Can you work these out from the drawing? Everything is in mm from the part's minimum corner. A direction names the side the tool comes from. Coordinates: 2 decimals unless noted, no trailing zeros. Loops run counter-clockwise (first coordinate to the right, second up) from the corner with the lowest first, then second, coordinate; pieces in that order, holes last. Notation, with made-up numbers: (66, -9) -> (124, -9) arc R28 cw to (124, 19) -> close; hole circle Ø8 at (70, -33.75). An arc over 180 degrees is marked (long way). One line per question, with ' | ' between items.
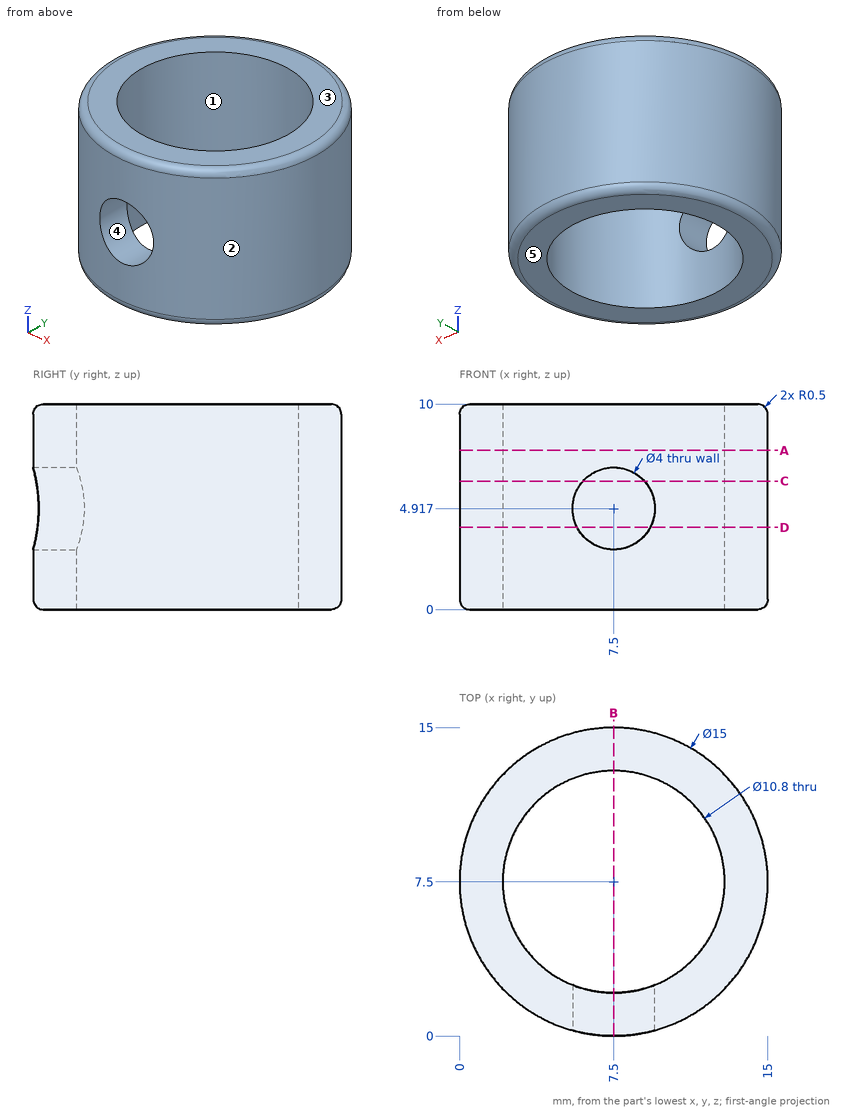
Q1. Imagine slicing it at C-C on z = 6.25. Write out the boundary of the cut face in (x, y), plus the area to 3 significant figures.
Values follow:
outline: (6.01, 0.15) -> (6.01, 2.31) arc R5.4 cw (long way) to (8.99, 2.31) -> (8.99, 0.15) arc R7.5 ccw (long way) to start | area: 78.8 mm2
Q2. Please list where these lines run through material, in increasing order: L1, parallel to Z at x = 7.5, y = 1.5; L2, parallel to Y at x = 7.5, z = 8; L3, parallel to X at y = 10.25, z = 1.25. Write a range as [from, to].
Values follow:
L1: z = [0, 2.92], [6.92, 10] | L2: y = [0, 2.1], [12.9, 15] | L3: x = [0.52, 2.85], [12.15, 14.48]
Q3. For pin 1 (6 mm diameter, centred on x = 3.5, z = 5.5, fed in from +Y); pin 2 (1 mm diameter, centred on y = 12, z = 4, fed in from +X); pin 3 (1 mm diameter, centred on y = 13.5, z = 5, fed in from +X), each with a flat end and sliding along its axis, tell me the tip position at first contact or that it passes through.
Values follow:
pin 1: stops at y = 14.93 | pin 2: stops at x = 13.84 | pin 3: stops at x = 12.6
Q4. Imagine slicing it at D-D on z = 4. Write out the boundary of the cut face in (x, y).
Values follow:
outline: (5.72, 0.21) -> (5.72, 2.4) arc R5.4 cw (long way) to (9.28, 2.4) -> (9.28, 0.21) arc R7.5 ccw (long way) to start
Q5. Imagine slicing it at B-B on x = 7.5. Give the number of separate pieces and of enclosed holes in the cut face, plus the area to 3 significant figures.
Values follow:
separate pieces: 3 | enclosed holes: 0 | area: 33.4 mm2
Q6. For the marked faces 4 and 5, which set-ups out of +Z, -Z, +X, -X, +Y, -Y let a thin tool reach every point of the face, with its end or its side?
Values follow:
face 4: -Y | face 5: -Z, +X, -X, +Y, -Y
Q7. We'd pull the mould along Y, two halves only. Please class the marked faces 1, 2 and 3: released by +Y, released by -Y, zero draft, split by the parting line, or undercut.
Values follow:
face 1: undercut | face 2: split by the parting line | face 3: zero draft
Q8. Imagine slicing it at A-A on z = 7.75. Write out the boundary of the cut face in (x, y), plus the area to 3 significant figures.
Values follow:
outline: circle Ø15 at (7.5, 7.5); hole circle Ø10.8 at (7.5, 7.5) | area: 85.1 mm2
